Source: CAD feature listing. Evaluate the final solid. Frame: model axes, mm. Face numbers are marked on the shaded views. Give positions to 0.01 mm unless a question says otherwise; leave off trailing zeros. Loops run counter-clockwise (first coordinate to the right, second up) from the corner with the lowest first, then second, coordinate; pieces in that order, holes last. Notation, with made-up numbers: (45.25, 79.5) - (50.25, 79.5) arc R16 ccw to (50.25, 88.5) - close; hole circle Ø1 at (-29.75, 64). An arc over 180 degrees is marked (long way). Put each result on its own line as item: value.
Autodesk Inventor part; units mm, degrees
ref_plane "YZ Plane" through (0, 0, 0) normal (1, 0, 0) x (0, 1, 0)
ref_plane "XZ Plane" through (0, 0, 0) normal (0, 1, 0) x (-1, 0, 0)
ref_plane "XY Plane" through (0, 0, 0) normal (0, 0, 1) x (1, 0, 0)
sketch "Sketch1" plane through (0, 0, 0) normal (0, 1, 0) x (-1, 0, 0)
  line L0 (0, 0) -> (69, 0)
  line L1 (69, 0) -> (69, -92)
  line L2 (69, -92) -> (0, -92)
  line L3 (0, -92) -> (0, 0)
  dimension "d0" = 69
  dimension "d1" = 92
extrude "Extrusion1" add sketch "Sketch1" along normal blind 1
sketch "Sketch2" plane through (0, 1, 0) normal (0, 1, 0) x (1, 0, 0)
  line L0 (-69, 0) -> (0, 0)
  line L1 (0, 0) -> (0, 92)
  line L2 (0, 92) -> (-69, 92)
  line L3 (-69, 92) -> (-69, 0)
  line L4 (-68, 1) -> (-1, 1)
  line L5 (-1, 1) -> (-1, 91)
  line L6 (-1, 91) -> (-68, 91)
  line L7 (-68, 91) -> (-68, 1)
  line L8 (-67.5, 1) -> (-67.5, 91)
  line L9 (-1.5, 1) -> (-1.5, 91)
  dimension "d4" = 1
  dimension "d5" = 0.5
  dimension "d6" = 0.5
extrude "Extrusion2" add sketch "Sketch2" along normal blind 5 contours L3 L2 L1 L0 | L7 L6 L8 L4 | L9 L6 L5 L4
sketch "Sketch3" plane through (0, 1, 0) normal (0, 1, 0) x (1, 0, 0)
  line L0 (-67.5, 91) -> (-67.5, 1)
  line L1 (-67.5, 1) -> (-1.5, 1)
  line L2 (-1.5, 1) -> (-1.5, 91)
  line L3 (-1.5, 91) -> (-67.5, 91)
  line L4 (-67.5, 1) -> (-1.5, 1)
  line L5 (-66.5, 1) -> (-66.5, 91)
  line L6 (-2.5, 1) -> (-2.5, 91)
  point P0 (0, 0)
  dimension "d9" = 1
  dimension "d10" = 1
extrude "Extrusion3" add sketch "Sketch3" along normal blind 12 contours L3 L5 L1 L0 | L3 L2 L1 L6
sketch "Sketch4" plane through (-1.5, 6, -91) normal (1, 0, 0) x (0, 0, -1)
  line L0 (-90, 0) -> (-90, 7)
  line L1 (-90, 4) -> (-90, 5)
  line L2 (0, 0) -> (0, 7)
  line L3 (-90, 7) -> (0, 7)
  line L4 (-60, 5) -> (-30, 5)
  line L5 (-30, 5) -> (-30, 4)
  line L6 (-30, 4) -> (-60, 4)
  line L7 (-60, 4) -> (-60, 5)
  line L8 (0, 0) -> (-90, 0)
  point P0 (-91, -6)
  dimension "d21" = 1
  dimension "d22" = 2
  dimension "d23" = 4
  dimension "d24" = 30
  dimension "d25" = 30
ref_plane "Work Plane1" through (-34.5, 0, 0) normal (1, 0, 0) x (0, 0, -1)
extrude "Extrusion5" add sketch "Sketch4" along normal blind 1 contours L4 L5 L6 L7
mirror "Mirror2" about plane through (-34.5, 0, 0) normal (1, 0, 0) of "Extrusion5"
properties part number "top1"
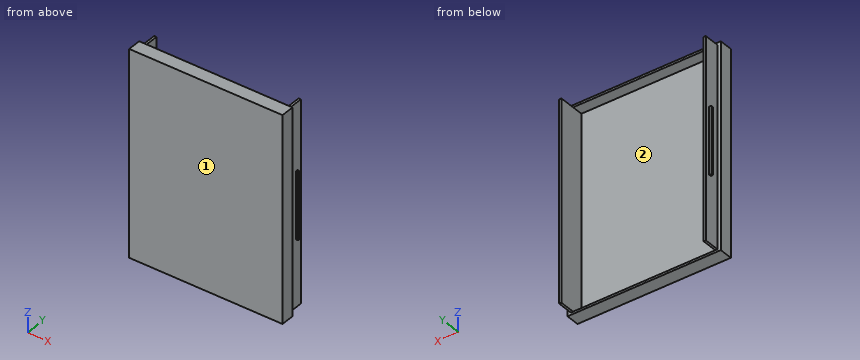
1) Mould query, pull axis Z, two halves, no side actions, for the marked faces 1 and 2. Classes: pulls with the +Z half, pulls with the -Z half, needs draft (parallel to the pull), parting line crosses it, or undercut.
Check result:
face 1: needs draft
face 2: undercut
2) Section query B-B, the plane z = -9. Output: boundary loops of the cut face in (x, y), plus the area to 3 significant figures.
Check result:
outline: (-69, 0) - (0, 0) - (0, 6) - (-1.5, 6) - (-1.5, 13) - (-2.5, 13) - (-2.5, 1) - (-66.5, 1) - (-66.5, 13) - (-67.5, 13) - (-67.5, 6) - (-69, 6) - close
area: 108 mm²
3) Pin query (flat end, axial travel): P1, Ø4, axis at x = -42.5, z = -71.5, coming from the +Y side; P2, Ø0.8, axis at x = -68, y = 10.5, coming from the -Z side; P3, Ø1.1, axis at x = -68, y = 10.5, coming from the +Z side. Return the tip coordinate at first contact, or that it passes through.
Check result:
P1: y = 1
P2: z = -61
P3: z = -1
4) Section query D-D, the plane x = -16. Output: boundary loops of the cut face in (y, z).
Check result:
outline: (0, -92) - (6, -92) - (6, -91) - (1, -91) - (1, -1) - (6, -1) - (6, 0) - (0, 0) - close
5) Section query A-A, the plane y = 8.75. Output: boundary loops of the cut face in (x, z).
Check result:
outline: (-67.5, -91) - (-66.5, -91) - (-66.5, -1) - (-67.5, -1) - close; (-2.5, -91) - (-1.5, -91) - (-1.5, -1) - (-2.5, -1) - close
6) Material intervals for line 1 along Z through (x, y) = (-65, 4.5); line 2 along X through (y, z) = (9.75, -21); line 3 along X through (y, z) = (2, -58.5), sorted ascending. Write a range as [from, to].
Check result:
line 1: [-92, -91], [-1, 0]
line 2: [-67.5, -66.5], [-2.5, -1.5]
line 3: [-69, -66.5], [-2.5, 0]
7) Section query C-C, the plane y = 2.5. Output: boundary loops of the cut face in (x, z), plus the area to 3 significant figures.
Check result:
outline: (-69, -92) - (0, -92) - (0, 0) - (-69, 0) - close; hole (-66.5, -91) - (-2.5, -91) - (-2.5, -1) - (-66.5, -1) - close
area: 588 mm²
